Geometry check sheet. Reference: the model listing, model coordinates, mm. Coordinates: 2 decimals unless noted, no trailing zeros. Write each loop counter-clockwise with the first axis right and the second up, starting at its lowest first coordinate (ties: lowest second). Pieces come first, ordered by that corner, then holes. Notation, with made-up numbers: M 20.5,40.25 L 53.5,40.25 A24 cw 53.5,57.25 Z; hole C 69.5,14 d9. An arc over 180 degrees is marked long. Answer as a JSON object with one key per item and string values. Group by question number.
```python
from build123d import *

# Parameters (mm, degrees)
SKETCH1_W           = 40
SKETCH1_H           = 40
SKETCH1_R           = 5.5
SKETCH1_R_2         = 1.5
SKETCH1_R_3         = 1.75
BOSS_EXTRUDE1_DEPTH = 5


with BuildPart() as part:
    # Sketch1 → Boss-Extrude1 (new body)
    with BuildSketch(Plane.XY):
        with Locations((0, 5)):
            Rectangle(SKETCH1_W, SKETCH1_H)
        Circle(SKETCH1_R, mode=Mode.SUBTRACT)
        with Locations((0, -8.5)):
            Circle(SKETCH1_R_2, mode=Mode.SUBTRACT)
        with Locations((0, 8.5)):
            Circle(SKETCH1_R_2, mode=Mode.SUBTRACT)
        with Locations((7.361215932, -4.25)):
            Circle(SKETCH1_R_2, mode=Mode.SUBTRACT)
        with Locations((-7.361215932, -4.25)):
            Circle(SKETCH1_R_2, mode=Mode.SUBTRACT)
        with Locations((-15, 20)):
            Circle(SKETCH1_R_3, mode=Mode.SUBTRACT)
        with Locations((-5, 20)):
            Circle(SKETCH1_R_3, mode=Mode.SUBTRACT)
        with Locations((5, 20)):
            Circle(SKETCH1_R_3, mode=Mode.SUBTRACT)
        with Locations((15, 20)):
            Circle(SKETCH1_R_3, mode=Mode.SUBTRACT)
    extrude(amount=BOSS_EXTRUDE1_DEPTH)


solid = part.part
```
1) Section check C-C (z = 3.1). State how many separate pieces and enclosed holes the cut face has, then the cut area to 3 significant figures.
2) Go/stop test with a flat-tipped pin: pin 1 Ø4 at (x, y) = (-15, 20) entering from +Z. Record where the tip stops, or that it passes through.
3) Section check A-A (x = 15). Record the cut outline in (y, z).
4) Draft check along Y on faces 1 (the cylindrical face through (5.863, -4.184, 2.465)), 2 (the flat face through (0, -15, 2)), 3 (the flat face through (-5, 5, 0)). Enter one of: +Y half, -Y half, draft (parallel to the pull), parting line (faces both ways), or undercut.
5) Section check B-B (y = 0). Record the cut outline in (x, z).
6) Section check D-D (x = 0). Record the cut outline in (y, z).
7) Material ranges on probe 1 along Y at (x, z) = (0, 2.45); probe 2 along X at (y, z) = (21, 3.2); probe 3 along Y at (x, z) = (-5, 1), recorded low to high. Write a range as [from, to].
Entries:
{
 "1": {"separate pieces": "1", "enclosed holes": "9", "area": "1,440 mm^2"},
 "2": {"pin 1": "z = 5"},
 "3": {"outline": "M -15,0 L 18.25,0 L 18.25,5 L -15,5 Z; M 21.75,0 L 25,0 L 25,5 L 21.75,5 Z"},
 "4": {"face 1": "undercut", "face 2": "-Y half", "face 3": "draft"},
 "5": {"outline": "M -20,0 L -5.5,0 L -5.5,5 L -20,5 Z; M 5.5,0 L 20,0 L 20,5 L 5.5,5 Z"},
 "6": {"outline": "M -15,0 L -10,0 L -10,5 L -15,5 Z; M -7,0 L -5.5,0 L -5.5,5 L -7,5 Z; M 5.5,0 L 7,0 L 7,5 L 5.5,5 Z; M 10,0 L 25,0 L 25,5 L 10,5 Z"},
 "7": {"probe 1": "[-15, -10], [-7, -5.5], [5.5, 7], [10, 25]", "probe 2": "[-20, -16.44], [-13.56, -6.44], [-3.56, 3.56], [6.44, 13.56], [16.44, 20]", "probe 3": "[-15, -2.29], [2.29, 18.25], [21.75, 25]"}
}
